Read the model definition and answer for the solid it produces. Units are mm, in the model's axes. Face numbers are marked on the shaded views. Give positions to 0.01 mm unless a question says otherwise; leave off trailing zeros. Loops run counter-clockwise (first coordinate to the right, second up) from the corner with the lowest first, then second, coordinate; pieces in that order, holes last. Notation, with made-up numbers: (17.25, 40.5) - (46.25, 40.5) arc R10 ccw to (46.25, 49.5) - close; hole circle Ø8 at (-21, 38). An arc over 180 degrees is marked (long way). Write item = value, one per line.
```python
from build123d import *

# Parameters (mm, degrees)
F0_W      = 150
F0_H      = 73
F1_DEPTH  = 7.873
F2_W      = 136
F2_H      = 63
F3_DEPTH  = 4.873
F4_W      = 2.5
F4_H      = 4.873
F5_DEPTH  = 73
F6_W      = 6.5
F6_H      = 0.623
F7_DEPTH  = 2.5
F8_R      = 1.25
F9_DEPTH  = 7.873
F10_R     = 1.25
F11_DEPTH = 7.873
F12_R     = 1.25
F13_DEPTH = 7.873
F14_R     = 1.25
F15_DEPTH = 7.873
F16_R     = 1.25
F17_DEPTH = 7.873
F18_R     = 1.25
F19_DEPTH = 7.873
F20_R     = 1.25
F21_DEPTH = 7.873
F22_R     = 1.25
F23_DEPTH = 7.873
F24_R     = 1.25
F25_DEPTH = 7.873
F26_R     = 1.25
F27_DEPTH = 7.873
F28_R     = 1.25
F29_DEPTH = 7.873
F30_R     = 1.25
F31_DEPTH = 7.873
F32_R     = 1.25
F33_DEPTH = 7.873
F34_R     = 1.25
F35_DEPTH = 7.873


with BuildPart() as f1:
    # F0 (on Top) → F1 (new body)
    with BuildSketch(Plane.XY):
        with Locations((75, 36.5)):
            Rectangle(F0_W, F0_H)
    extrude(amount=F1_DEPTH)

    # F2 (on Top) → F3 (cut)
    with BuildSketch(Plane.XY):
        with Locations((75, 36.5)):
            Rectangle(F2_W, F2_H)
    extrude(amount=F3_DEPTH, mode=Mode.SUBTRACT)

    # F4 (on Front) → F5 (join)
    with BuildSketch(Plane.XZ):
        with Locations((75, 2.4365)):
            Rectangle(F4_W, F4_H)
    extrude(amount=-F5_DEPTH)

    # F6 (on face) → F7 (cut)
    with BuildSketch(Plane(origin=(73.75, 0, 0), x_dir=(0, -1, 0), z_dir=(-1, 0, 0))):
        with Locations((-36.5, 0.3115)):
            Rectangle(F6_W, F6_H)
    extrude(amount=-F7_DEPTH, mode=Mode.SUBTRACT)

    # F8 (on face) → F9 (cut)
    with BuildSketch(Plane.XY.offset(7.873)):
        with Locations((2.5, 2.5)):
            Circle(F8_R)
    extrude(amount=-F9_DEPTH, mode=Mode.SUBTRACT)

    # F10 (on face) → F11 (cut)
    with BuildSketch(Plane.XY.offset(7.873)):
        with Locations((18, 2.5)):
            Circle(F10_R)
    extrude(amount=-F11_DEPTH, mode=Mode.SUBTRACT)

    # F12 (on face) → F13 (cut)
    with BuildSketch(Plane.XY.offset(7.873)):
        with Locations((34.5, 2.5)):
            Circle(F12_R)
    extrude(amount=-F13_DEPTH, mode=Mode.SUBTRACT)

    # F14 (on face) → F15 (cut)
    with BuildSketch(Plane.XY.offset(7.873)):
        with Locations((51, 2.5)):
            Circle(F14_R)
    extrude(amount=-F15_DEPTH, mode=Mode.SUBTRACT)

    # F16 (on face) → F17 (cut)
    with BuildSketch(Plane.XY.offset(7.873)):
        with Locations((67.5, 2.5)):
            Circle(F16_R)
    extrude(amount=-F17_DEPTH, mode=Mode.SUBTRACT)

    # F18 (on face) → F19 (cut)
    with BuildSketch(Plane.XY.offset(7.873)):
        with Locations((82.5, 2.5)):
            Circle(F18_R)
    extrude(amount=-F19_DEPTH, mode=Mode.SUBTRACT)

    # F20 (on face) → F21 (cut)
    with BuildSketch(Plane.XY.offset(7.873)):
        with Locations((99, 2.5)):
            Circle(F20_R)
    extrude(amount=-F21_DEPTH, mode=Mode.SUBTRACT)

    # F22 (on face) → F23 (cut)
    with BuildSketch(Plane.XY.offset(7.873)):
        with Locations((115.5, 2.5)):
            Circle(F22_R)
    extrude(amount=-F23_DEPTH, mode=Mode.SUBTRACT)

    # F24 (on face) → F25 (cut)
    with BuildSketch(Plane.XY.offset(7.873)):
        with Locations((132, 2.5)):
            Circle(F24_R)
    extrude(amount=-F25_DEPTH, mode=Mode.SUBTRACT)

    # F26 (on face) → F27 (cut)
    with BuildSketch(Plane.XY.offset(7.873)):
        with Locations((147.5, 2.5)):
            Circle(F26_R)
    extrude(amount=-F27_DEPTH, mode=Mode.SUBTRACT)

    # F28 (on face) → F29 (cut)
    with BuildSketch(Plane.XY.offset(7.873)):
        with Locations((2.5, 22)):
            Circle(F28_R)
    extrude(amount=-F29_DEPTH, mode=Mode.SUBTRACT)

    # F30 (on face) → F31 (cut)
    with BuildSketch(Plane.XY.offset(7.873)):
        with Locations((147.5, 22)):
            Circle(F30_R)
    extrude(amount=-F31_DEPTH, mode=Mode.SUBTRACT)

    # F32 (on face) → F33 (cut)
    with BuildSketch(Plane.XY.offset(7.873)):
        with Locations((147.5, 38.5)):
            Circle(F32_R)
    extrude(amount=-F33_DEPTH, mode=Mode.SUBTRACT)

    # F34 (on face) → F35 (cut)
    with BuildSketch(Plane.XY.offset(7.873)):
        with Locations((2.5, 38.5)):
            Circle(F34_R)
    extrude(amount=-F35_DEPTH, mode=Mode.SUBTRACT)


solid = f1.part
```
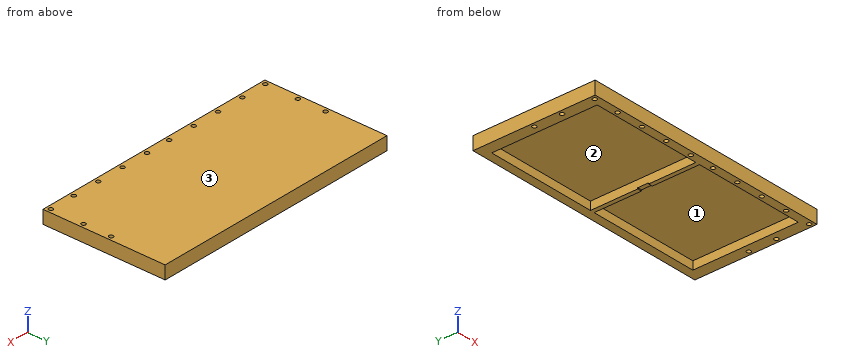
1) Find the intervals of material crossed by probe 1 along Y at (x, z) = (147.5, 5.5); probe 2 along Y at (x, z) = (99, 2.75); probe 3 along X at (y, z) = (47, 4.75), in increasing order.
Output:
probe_1 = 0 to 1.25, 3.75 to 20.75, 23.25 to 37.25, 39.75 to 73
probe_2 = 0 to 1.25, 3.75 to 5, 68 to 73
probe_3 = 0 to 7, 73.75 to 76.25, 143 to 150
2) This flat-tipped pin is pushed along its axis until it touches: P1, Ø2, axis at x = 19, y = 16.5, coming from the -Z side. Where does it stop, or does it pass through?
Output:
P1 = 4.87
3) A cutting plane is placed at B-B on y = 50.5. Determine the outline of the cut face in (x, z), then the cut area to 3 significant figures.
Output:
outline = (0, 0) - (7, 0) - (7, 4.87) - (73.75, 4.87) - (73.75, 0) - (76.25, 0) - (76.25, 4.87) - (143, 4.87) - (143, 0) - (150, 0) - (150, 7.87) - (0, 7.87) - close
area = 530 mm²
4) A cutting plane is placed at A-A on x = 10.5. Determine the outline of the cut face in (y, z).
Output:
outline = (0, 0) - (5, 0) - (5, 4.87) - (68, 4.87) - (68, 0) - (73, 0) - (73, 7.87) - (0, 7.87) - close
5) The mould has two halves that part along X. Classify the marked faces 1, 2 and 3: pulls with the +X half, pulls with the -X half, needs draft (parallel to the pull), parting line crosses it, or undercut.
Output:
face_1 = undercut
face_2 = undercut
face_3 = needs draft
